Geometry check sheet. Reference: the model listing, model coordinates, mm. Coordinates: 2 decimals unless noted, no trailing zeros. Order: outer loops, then holes, each group sorted by start corner. A loop starts at its lowest first (then second) coordinate and runs counter-clockwise, first axis right, second up. Notation, with made-up numbers: (-39, 11.25) - (16, 11.25) arc R18 cw to (16, 16.25) - close; hole circle Ø4 at (20, -25.5). An arc over 180 degrees is marked (long way). Put each result on its own line as item: value.
from build123d import *

# Parameters (mm, degrees)
BOSS_EXTRUDE1_DEPTH            = 19.05
F_7_0_201_DIAMETER_HOLE1_D     = 5.1054
F_7_0_201_DIAMETER_HOLE1_DEPTH = 25.4


with BuildPart() as part:
    # Sketch2 → Boss-Extrude1 (new body)
    with BuildSketch(Plane.XY):
        Polygon((0, 0), (0, 34.992683716), (-56.000000014, 0), align=None)
    extrude(amount=BOSS_EXTRUDE1_DEPTH)

    # #7 (0.201) Diameter Hole1
    with Locations(Plane(origin=(-15.725607894, 25.166233303, 0), x_dir=(0.8480480961564308, 0.5299192642331972, 0), z_dir=(-0.5299192642331972, 0.848048096156431, 0))):
        with Locations((-35.431702792, -9.525), (9.018297208, -9.525)):
            Hole(F_7_0_201_DIAMETER_HOLE1_D / 2, depth=F_7_0_201_DIAMETER_HOLE1_DEPTH)


solid = part.part
Q1. Section check C-C on z = 5. Record the boundary of the cut face in (x, y), then the cut area to 3 significant figures.
Answer block:
outline: (-56, 0) - (0, 0) - (0, 34.99) - close
area: 980 mm^2
Q2. Thickness scan on L1, parallel to X at y = 4, z = 10.75; L2, parallel to X at y = 32.5, z = 2; L3, parallel to X at y = 9, z = 10.5. Record the ranges inside material, lowest first. Write a range as [from, to].
Answer block:
L1: x = [-49.6, -46.92], [-41.64, 0]
L2: x = [-3.99, 0]
L3: x = [-41.6, 0]
Q3. Section check D-D on y = 11. Record the boundary of the cut face in (x, z).
Answer block:
outline: (-38.4, 0) - (0, 0) - (0, 19.05) - (-38.4, 19.05) - close
Q4. Depth check by flat-ended pin: pin 1 Ø6 at (x, z) = (-30.5, 10) entering from +Y; pin 2 Ø5 at (x, z) = (-15, 14.5) entering from +Y; pin 3 Ø1.5 at (y, z) = (19.5, 15) entering from -X. Enter the tip coordinate at first touch or a pass-through.
Answer block:
pin 1: stops at y = 17.81
pin 2: stops at y = 27.18
pin 3: stops at x = -25.99
Q5. Section check A-A on z = 8. Record the boundary of the cut face in (x, y).
Answer block:
outline: (-56, 0) - (-44.19, 0) - (-47.51, 5.31) - close; (-44.04, 7.48) - (-39.37, 0) - (0, 0) - (0, 13.16) - (-9.81, 28.86) - close; (-6.34, 31.03) - (0, 20.88) - (0, 34.99) - close
Q6. Draft check along Z on faces 1 (the cylindrical face through (-41.664, 4.626, 9.413)), 2 (the flat face through (-16, 10, 19.05)), 3 (the flat face through (0, 17, 14)). Enter one of: pulls with the +Z half, pulls with the -Z half, needs draft (parallel to the pull), parting line crosses it, or undercut.
Answer block:
face 1: undercut
face 2: pulls with the +Z half
face 3: needs draft
Q7. Section check B-B on x = -19. Record the boundary of the cut face in (y, z), then the cut area to 3 significant figures.
Answer block:
outline: (0, 0) - (23.12, 0) - (23.12, 19.05) - (0, 19.05) - close
area: 440 mm^2
